Can you work these out from the model? Positions are in its coordinate system, mm. Face numbers are marked on the shaded views. A direction names the side the tool comes from. Coordinates: 2 decimals unless noted, no trailing zeros. Write each loop counter-clockwise with the first axis right and the second up, starting at its lowest first coordinate (ties: lowest second). Pieces come first, ordered by that corner, then holes.
```python
from build123d import *

# Parameters (mm, degrees)
SKETCH_1_R               = 60
EXTRUDE_1_DEPTH          = 30
SKETCH_2_R               = 1.5
CUT_EXTRUDE_1_DEPTH      = 5
PATTERN_CIRCULAR_1_COUNT = 10
SKETCH_3_W               = 40
SKETCH_3_H               = 20
EXTRUDE_2_DEPTH          = 30
SKETCH_5_R               = 2.5
EXTRUDE_4_DEPTH          = 1
SKETCH_7_R               = 2.5
CUT_EXTRUDE_2_DEPTH      = 1


with BuildPart() as part:
    # 草图1 → 凸台-拉伸1 (new body)
    with BuildSketch(Plane(origin=(0, 0, 0), x_dir=(1, 0, 0), z_dir=(0, 1, 0))):
        with Locations(Location((0, 0, 0), (0, 0, 270))):
            Circle(SKETCH_1_R)
    extrude(amount=EXTRUDE_1_DEPTH)

    # 草图2 → 切除-拉伸1 (cut)
    with BuildSketch(Plane(origin=(0, 30, 0), x_dir=(1, 0, 0), z_dir=(0, 1, 0))):
        with Locations(Location((55, 0, 0), (0, 0, 270))):
            Circle(SKETCH_2_R)
    cut_extrude_1 = extrude(amount=-CUT_EXTRUDE_1_DEPTH, mode=Mode.SUBTRACT)

    # 阵列(圆周)1: 切除-拉伸1 ×10 about axis
    pattern_circular_1_axis = Axis((0, 0, 0), (0, 1, 0))
    for i in range(1, PATTERN_CIRCULAR_1_COUNT):
        add(cut_extrude_1.rotate(pattern_circular_1_axis, i * 360 / PATTERN_CIRCULAR_1_COUNT), mode=Mode.SUBTRACT)

    # 草图3 → 凸台-拉伸2 (add)
    with BuildSketch(Plane(origin=(0, 30, 0), x_dir=(1, 0, 0), z_dir=(0, 1, 0))):
        Rectangle(SKETCH_3_W, SKETCH_3_H)
    extrude(amount=EXTRUDE_2_DEPTH)

    # 草图5 → 凸台-拉伸4 (add)
    with BuildSketch(Plane(origin=(0, 30, 0), x_dir=(1, 0, 0), z_dir=(0, 1, 0))):
        with Locations(Location((-44.495934691, 32.328188876, 0), (0, 0, 270))):
            Circle(SKETCH_5_R)
        with Locations(Location((44.495934691, -32.328188876, 0), (0, 0, 270))):
            Circle(SKETCH_5_R)
        with Locations(Location((44.495934691, 32.328188876, 0), (0, 0, 270))):
            Circle(SKETCH_5_R)
        with Locations(Location((-44.495934691, -32.328188876, 0), (0, 0, 270))):
            Circle(SKETCH_5_R)
    extrude(amount=EXTRUDE_4_DEPTH)

    # 草图7 → 切除-拉伸2 (cut)
    with BuildSketch(Plane.XZ):
        with Locations(Location((0, 0, 0), (0, 0, 270))):
            Circle(SKETCH_7_R)
    extrude(amount=-CUT_EXTRUDE_2_DEPTH, mode=Mode.SUBTRACT)


solid = part.part
```
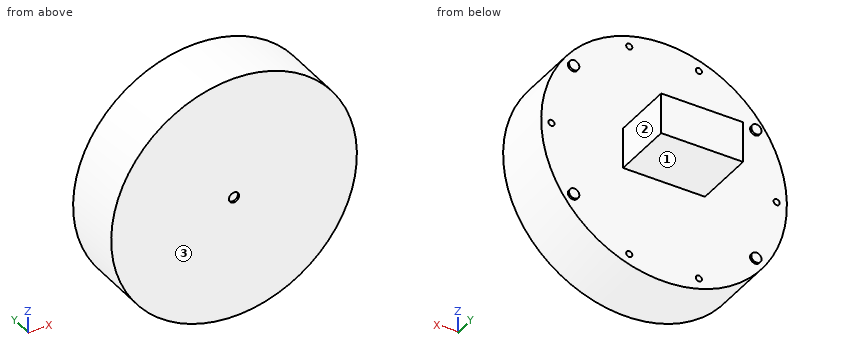
1. If I drill on L1, parallel to Y at x = 46, z = 24.5; L2, parallel to Z at x = -55, y = 26.75; L3, parallel to Z at x = -14, y = 38.5, over which ranges is the centre line in solid material (lowest first)?
2. If we section it at C-C, the plane y = 41.5: List the corners of the cut face in (x, z) for me, plus the area to 3 significant figures.
3. Which directions (+Z, -Z, +X, -X, +Y, -Y) give clear straight access to the entire face, cutting with the end or side of a thin tool? Please do the marked faces 1, 2 and 3.
4. I'm going to push flat-ended pins straight in: P1, Ø12, axis at y = 45.5, z = 12.5, coming from the +X side; P2, Ø1.5, axis at x = -17, z = -52, coming from the +Y side; P3, Ø12, axis at x = 27, z = -29.5, coming from the +Y side. Where does each tip first touch, or does it pass through?
5. If we section it at D-D, the plane x = -55: List the corners of the cut face in (y, z) for me, plus the area to 3 significant figures.
6. If we section it at B-B, the plane z = 0: List the corners of the cut face in (x, y) for me, plus the area to 4 significant figures.
7. If we section it at A-A, the plane x = 0: List the corners of the cut face in (y, z) for me, plus the area to 4 significant figures.
Answers:
1. L1: y = 0 to 30
1. L2: z = -23.98 to -1.5, 1.5 to 23.98
1. L3: z = -10 to 10
2. outline: (-20, -10) - (20, -10) - (20, 10) - (-20, 10) - close
2. area: 800 mm2
3. face 1: -Z, +X, -X, +Y
3. face 2: +Z, -Z, +X, +Y
3. face 3: +Z, -Z, +X, -X, -Y
4. P1: stops at x = 20
4. P2: stops at y = 25
4. P3: stops at y = 30
5. outline: (0, -23.98) - (30, -23.98) - (30, -1.5) - (25, -1.5) - (25, 1.5) - (30, 1.5) - (30, 23.98) - (0, 23.98) - close
5. area: 1,420 mm2
6. outline: (-60, 0) - (-2.5, 0) - (-2.5, 1) - (2.5, 1) - (2.5, 0) - (60, 0) - (60, 30) - (56.5, 30) - (56.5, 25) - (53.5, 25) - (53.5, 30) - (20, 30) - (20, 60) - (-20, 60) - (-20, 30) - (-53.5, 30) - (-53.5, 25) - (-56.5, 25) - (-56.5, 30) - (-60, 30) - close
6. area: 4,765 mm2
7. outline: (0, -60) - (30, -60) - (30, -10) - (60, -10) - (60, 10) - (30, 10) - (30, 60) - (0, 60) - (0, 2.5) - (1, 2.5) - (1, -2.5) - (0, -2.5) - close
7. area: 4,195 mm2
